Design review of the part built by this model. Coordinates are the model's own, in mm. Face numbers are marked on the shaded views. A direction names the side the tool comes from. Coordinates: 2 decimals unless noted, no trailing zeros. Loops run counter-clockwise (first coordinate to the right, second up) from the corner with the lowest first, then second, coordinate; pieces in that order, holes last. Notation, with made-up numbers: (-14, -11) -> (14, -11) arc R26 cw to (14, 5) -> close; hole circle Ø11 at (-21.5, 12.25). An arc over 180 degrees is marked (long way). Answer in a Markdown table with one row per item.
```python
from build123d import *

# Parameters (mm, degrees)
SKETCH_1_R      = 3.5775
SKETCH_1_R_2    = 0.36
SKETCH_1_R_3    = 0.19875
EXTRUDE_2_DEPTH = 0.159
EXTRUDE_START   = 0.3975
SKETCH_1_6_R    = 0.19875
SKETCH_1_6_R_2  = 0.36
EXTRUDE_3_DEPTH = 0.3975
SCALE_3_SCALE   = 25


with BuildPart() as part:
    # Sketch 1 → Extrude 2 (new body)
    # profile 1 of 3: a face of its own
    with BuildSketch(Plane.XY):
        Circle(SKETCH_1_R)
        with Locations((-3.18, 0)):
            Circle(SKETCH_1_R_2, mode=Mode.SUBTRACT)
        with BuildLine():
            ThreePointArc((-0.770493853, -0.756795363), (1.069529145, 0.150024692), (-0.948975285, 0.515602472))
            ThreePointArc((-0.948975285, 0.515602472), (-0.794802322, -0.111488288), (-0.770493853, -0.756795363))
        make_face(mode=Mode.SUBTRACT)
    # profile 2 of 3: a face of its own
    with BuildSketch(Plane.XY):
        with BuildLine():
            ThreePointArc((-0.770493853, -0.756795363), (-0.794802322, -0.111488288), (-0.948975285, 0.515602472))
            ThreePointArc((-0.948975285, 0.515602472), (1.069529145, 0.150024692), (-0.770493853, -0.756795363))
        make_face()
        Circle(SKETCH_1_R_3, mode=Mode.SUBTRACT)
    # profile 3 of 3: a face of its own
    with BuildSketch(Plane.XY):
        with Locations((-3.18, 0)):
            Circle(SKETCH_1_R_2)
    extrude(amount=-EXTRUDE_2_DEPTH)

    # Sketch 1_6 → Extrude 3 (add)
    # profile 1 of 2: a face of its own
    with BuildSketch(Plane.XY.offset(EXTRUDE_START)):
        with BuildLine():
            ThreePointArc((-0.770493853, -0.756795363), (-0.794802322, -0.111488288), (-0.948975285, 0.515602472))
            ThreePointArc((-0.948975285, 0.515602472), (1.069529145, 0.150024692), (-0.770493853, -0.756795363))
        make_face()
        Circle(SKETCH_1_6_R, mode=Mode.SUBTRACT)
    # profile 2 of 2: a face of its own
    with BuildSketch(Plane.XY.offset(EXTRUDE_START)):
        with Locations((-3.18, 0)):
            Circle(SKETCH_1_6_R_2)
    extrude(amount=-EXTRUDE_3_DEPTH)


with BuildPart() as part_1:
    # Scale 3: scaled about (-0.054347158, 0.00157736, -0.027262254)
    add(part.part.scale(SCALE_3_SCALE).moved(Location((1.304331792, -0.03785664, 0.654294096))))


solid = part_1.part
```
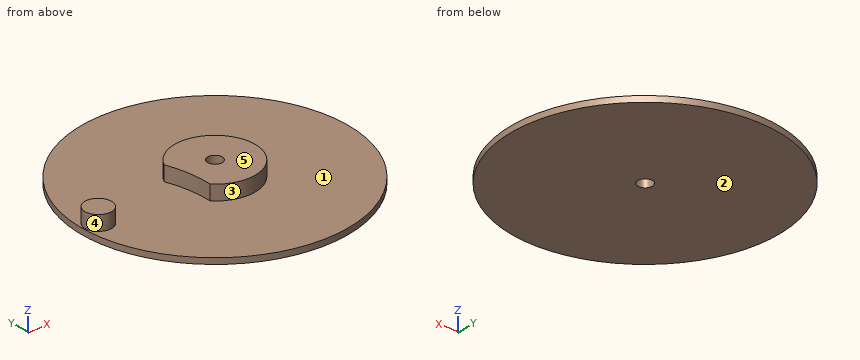
(1) For pin 1 (13 mm diameter, centred on x = 1.3, y = -0.04, fed in from +Z); pin 2 (2 mm diameter, centred on y = 46, z = -1, fed in from -X); pin 3 (4 mm diameter, centred on x = 29.5, z = -1.5, fed in from -Y); pin 4 (4 mm diameter, centred on y = 24, z = 6, fed in from +X), all flat-tipped, find the tip position at first contact; note any pin that passes through.
Evaluation:
| item | result |
|---|---|
| pin 1 | stops at z = 10.59 |
| pin 2 | stops at x = -75.97 |
| pin 3 | stops at y = -85.55 |
| pin 4 | stops at x = 16.9 |
(2) To check wall thickness, follow probe 1 along X at (y, z) = (3, 8.25); probe 2 along X at (y, z) = (-2.5, 7.5); probe 3 along Z at (x, y) = (26.5, 40). State the ranges of each line that lie inside material, in increasing order.
Evaluation:
| item | result |
|---|---|
| probe 1 | x = -86.67 to -69.72, -19.61 to -2.63, 5.24 to 28.13 |
| probe 2 | x = -86.85 to -69.54, -18.61 to -3.01, 5.62 to 28.19 |
| probe 3 | z = -3.32 to 0.65 |
(3) Take a section at A-A on z = 7. Give the boundary of the cut face in (x, y).
Evaluation:
| item | result |
|---|---|
| outline | circle Ø18 at (-78.2, -0.04); (-22.42, 12.85) arc R79.5 cw to (-17.96, -18.96) arc R27 ccw (long way) to start; hole circle Ø9.94 at (1.3, -0.04) |
(4) Take a section at D-D on y = 36.5. Give the boundary of the cut face in (x, z).
Evaluation:
| item | result |
|---|---|
| outline | (-80.33, -3.32) -> (82.94, -3.32) -> (82.94, 0.65) -> (-80.33, 0.65) -> close |
(5) Tool access review of the marked faces 1 and 2: name each direction out of +Z, -Z, +X, -X, +Y, -Y from which nothing blocks a thin tool from reaching the whole face with its end or side.
Evaluation:
| item | result |
|---|---|
| face 1 | +Z |
| face 2 | -Z, +X, -X, +Y, -Y |
(6) Take a section at C-C on x = 10. Give the boundary of the cut face in (y, z), and give its area (3 significant figures).
Evaluation:
| item | result |
|---|---|
| outline | (-89.05, -3.32) -> (88.98, -3.32) -> (88.98, 0.65) -> (25.52, 0.65) -> (25.52, 10.59) -> (-25.6, 10.59) -> (-25.6, 0.65) -> (-89.05, 0.65) -> close |
| area | 1,220 mm² |
(7) Draft analysis for pull direction X (two halves, no side actions). For the marked faces 3, 4 and 5, state which applies: pulls with the +X half, pulls with the -X half, needs draft (parallel to the pull), parting line crosses it, or undercut.
Evaluation:
| item | result |
|---|---|
| face 3 | parting line crosses it |
| face 4 | undercut |
| face 5 | needs draft |
(8) Take a section at B-B on x = -10. Give the boundary of the cut face in (y, z).
Evaluation:
| item | result |
|---|---|
| outline | (-88.76, -3.32) -> (88.68, -3.32) -> (88.68, 0.65) -> (24.48, 0.65) -> (24.48, 10.59) -> (-24.56, 10.59) -> (-24.56, 0.65) -> (-88.76, 0.65) -> close |
